from build123d import *

# Parameters (mm, degrees)
SALIENTE_EXTRUIR1_DEPTH = 20
VACIADO1_T              = 1
CORTAR_EXTRUIR1_REACH   = 143.043
CROQUIS2_W              = 47.810995816
CROQUIS2_H              = 20
CORTAR_EXTRUIR7_REACH   = 142.243
CROQUIS10_W             = 25
CROQUIS10_H             = 32
CORTAR_EXTRUIR8_REACH   = 142.83
CROQUIS11_W             = 31.5
CROQUIS11_H             = 8
SALIENTE_EXTRUIR2_DEPTH = 12
CORTAR_EXTRUIR9_REACH   = 142.389
CROQUIS13_W             = 42
CROQUIS13_H             = 45


with BuildPart() as part:
    # Croquis1 → Saliente-Extruir1 (new body)
    with BuildSketch(Plane(origin=(0, 0, 0), x_dir=(1, 0, 0), z_dir=(0, 1, 0))):
        Polygon((0, 16.5), (17, 0), (64, 0), (81, 16.5), (81, 94.5), (64, 111), (17, 111), (0, 94.5), align=None)
    extrude(amount=SALIENTE_EXTRUIR1_DEPTH)

    # Vaciado1
    vaciado1_openings = [part.faces().sort_by_distance(p)[0] for p in [
        (40.5, 20, -55.5),
    ]]
    offset(amount=VACIADO1_T, openings=vaciado1_openings, kind=Kind.INTERSECTION)

    # Croquis2 → Cortar-Extruir1 (cut, up to next)
    with BuildSketch(Plane.XY.offset(1), mode=Mode.PRIVATE) as cortar_extruir1_sk1:
        with Locations((40.5, 10)):
            Rectangle(CROQUIS2_W, CROQUIS2_H)
    cortar_extruir1_tool1 = extrude(cortar_extruir1_sk1.sketch, amount=-CORTAR_EXTRUIR1_REACH, mode=Mode.PRIVATE) & part.part
    add(cortar_extruir1_tool1.solids().sort_by_distance((40.5, 10, 1))[0], mode=Mode.SUBTRACT)

    # Croquis10 → Cortar-Extruir7 (cut, up to next)
    with BuildSketch(Plane(origin=(0, 0, 0), x_dir=(1, 0, 0), z_dir=(0, 1, 0)), mode=Mode.PRIVATE) as cortar_extruir7_sk1:
        with Locations((40.5, 15)):
            Rectangle(CROQUIS10_W, CROQUIS10_H)
    cortar_extruir7_tool1 = extrude(cortar_extruir7_sk1.sketch, amount=-CORTAR_EXTRUIR7_REACH, mode=Mode.PRIVATE) & part.part
    add(cortar_extruir7_tool1.solids().sort_by_distance((40.5, 0, -15))[0], mode=Mode.SUBTRACT)

    # Croquis11 → Cortar-Extruir8 (cut, up to next)
    with BuildSketch(Plane.ZY.offset(1), mode=Mode.PRIVATE) as cortar_extruir8_sk1:
        with Locations((-33.827016736, 16)):
            Rectangle(CROQUIS11_W, CROQUIS11_H)
    cortar_extruir8_tool1 = extrude(cortar_extruir8_sk1.sketch, amount=-CORTAR_EXTRUIR8_REACH, mode=Mode.PRIVATE) & part.part
    add(cortar_extruir8_tool1.solids().sort_by_distance((-1, 16, -33.827017))[0], mode=Mode.SUBTRACT)

    # Croquis12 → Saliente-Extruir2 (add)
    with BuildSketch(Plane(origin=(0, 0, 0), x_dir=(1, 0, 0), z_dir=(0, 1, 0))):
        Polygon((16.594502092, 0.393571499), (17.290977469, 1.111152191), (1, 16.922983264), (1, 94.077016736), (17.405497908, 110), (63.594502092, 110), (80, 94.077016736), (80, 16.922983264), (63.709022531, 1.111152191), (64.405497908, 0.393571499), (81, 16.5), (81, 94.5), (64, 111), (17, 111), (0, 94.5), (0, 16.5), align=None)
    extrude(amount=SALIENTE_EXTRUIR2_DEPTH)

    # Croquis13 → Cortar-Extruir9 (cut, up to next)
    with BuildSketch(Plane.XZ.offset(1), mode=Mode.PRIVATE) as cortar_extruir9_sk1:
        with Locations((40.5, -74.5)):
            Rectangle(CROQUIS13_W, CROQUIS13_H)
    cortar_extruir9_tool1 = extrude(cortar_extruir9_sk1.sketch, amount=-CORTAR_EXTRUIR9_REACH, mode=Mode.PRIVATE) & part.part
    add(cortar_extruir9_tool1.solids().sort_by_distance((40.5, -1, -74.5))[0], mode=Mode.SUBTRACT)


solid = part.part
Model file for the job. Use its own axes, mm. A direction names the side the tool comes from. Give positions to 0.01 mm unless a question says otherwise; leave off trailing zeros. Order: outer loops, then holes, each group sorted by start corner. A loop starts at its lowest first (then second) coordinate and runs counter-clockwise, first axis right, second up. Notation, with made-up numbers: M 47.25,63 L 70.25,63 A29 cw 70.25,93 Z; hole C -31,32.5 d6. An arc over 180 degrees is marked long. Put each result on its own line as item: value. Start each with the question number.
(1) Band-saw the part on A-A on x = 37.5. Give the cut face in (y, z).
(2) Band-saw the part on D-D on y = 4. Give the cut face in (x, z), then the cut area to 3 significant figures.
(3) Band-saw the part on C-C on z = -41.5. Give the cut face in (x, y), then the cut area to 3 significant figures.
(4) Pull direction X, two halves, no side cores. Call faces 4 (the face through (80, 6, -56)), 5 (the face through (41, 9, -112)), 6 (the face through (-1, 7, -56)): released by +X, released by -X, zero draft, split by the parting line, or undercut.
(5) Tool access for faces 1 (the face through (8.18, 15.94, -8.56)), 2 (the face through (7.67, 9.35, -7.66)), 3 (the face through (40, 6, -110)): list every direction of +Z, -Z, +X, -X, +Y, -Y with a clear straight run to the whole face (end or side of a thin tool).
(6) Pin check, flat tips, straight feed: pin 1 Ø1.1 at (x, y) = (38.5, -0.5) entering from +Z; pin 2 Ø10 at (x, y) = (46.5, 16) entering from +Z; pin 3 Ø3 at (x, z) = (14, -47.5) entering from +Y; pin 4 Ø4 at (x, z) = (21, -95.5) entering from -Y. Stop position of each tip, or through.
(7) Band-saw the part on B-B on y = 13.5. Give the cut face in (x, z), then the cut area to 3 significant figures.
(8) Drill centre lines: L1, parallel to X at y = 10.75, z = -77.5; L2, parallel to X at y = 17.5, z = -74; L3, parallel to Z at x = 44, y = 5.75. Where is each one in solid material? Low to high. Write a range as [from, to].
Results below:
1. outline: M -1,-112 L 20,-112 L 20,-111 L 12,-111 L 12,-110 L 0,-110 L 0,-97 L -1,-97 Z; M -1,-52 L 0,-52 L 0,-31 L -1,-31 Z
2. outline: M -1,-94.92 L 16.59,-112 L 64.41,-112 L 82,-94.92 L 82,-16.08 L 64.41,1 L 64.41,-0.39 L 63.71,-1.11 L 80,-16.92 L 80,-94.08 L 63.59,-110 L 17.41,-110 L 1,-94.08 L 1,-16.92 L 17.29,-1.11 L 16.59,-0.39 L 16.59,1 L -1,-16.08 Z
2. area: 594 mm2
3. outline: M -1,-1 L 82,-1 L 82,20 L 81,20 L 81,12 L 80,12 L 80,0 L 1,0 L 1,12 L -1,12 Z
3. area: 139 mm2
4. face 4: undercut
4. face 5: zero draft
4. face 6: released by -X
5. face 1: +Y
5. face 2: +Z, -X, +Y, -Y
5. face 3: +Z, +Y
6. pin 1: stops at z = -31
6. pin 2: stops at z = -110
6. pin 3: stops at y = 0
6. pin 4: stops at y = -1
7. outline: M -1,-94.92 L 16.59,-112 L 64.41,-112 L 82,-94.92 L 82,-16.08 L 64.41,1 L 64.41,-0.39 L 81,-16.5 L 81,-94.5 L 64,-111 L 17,-111 L 0,-94.5 L 0,-49.58 L -1,-49.58 Z; M -1,-18.08 L 0,-18.08 L 0,-16.5 L 16.59,-0.39 L 16.59,1 L -1,-16.08 Z
7. area: 269 mm2
8. L1: x = [-1, 1], [80, 82]
8. L2: x = [-1, 0], [81, 82]
8. L3: z = [-112, -110]
